The figure shows three views and two pictorial views of one solid part (mm, origin at its lowest corner). Answer the questions. A direction names the side the tool comes from. Give positions to 0.01 mm unless a question says otherwise; leave off trailing zeros. Write each loop counter-clockwise with the first axis right and the second up, starting at its lowest first coordinate (ties: lowest second). Pieces come first, ordered by that corner, then holes. Notation, with made-up numbers: (16.5, 81) -> (62.5, 81) arc R31 cw to (62.5, 110) -> close; hole circle Ø2 at (60, 51.5). An arc over 180 degrees is marked (long way). Write each question's results on one line, items separated by ' | '. Start each with the question number.
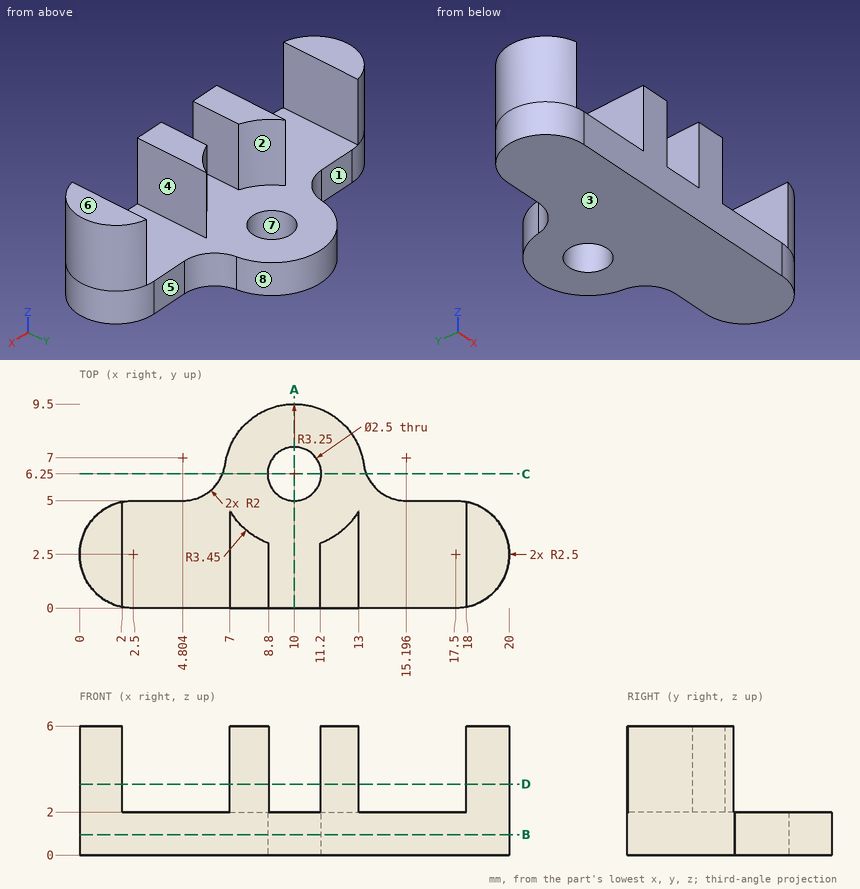
1. The mould has two halves that part along X. Classify the marked faces 6, 7 and 8: pulls with the +X half, pulls with the -X half, needs draft (parallel to the pull), parting line crosses it, or undercut.
2. A tool of negligible diameter and unlimited length cuts with its end or side. For the marked faces 1, 2, 3, 4 and 5, from which of +Z, -Z, +X, -X, +Y, -Y can it reach the whole face along a straight path? Write none if from no direction.
3. Section B-B (z = 0.95) is taken. Write down the section's boundary in (x, y).
4. Each of these flat-tipped pins is pushed along its axis until it touches: pin 1 Ø2.5 at (y, z) = (1, 4) entering from +X; pin 2 Ø1.6 at (x, z) = (16, 1.5) entering from +Y; pin 3 Ø1.2 at (y, z) = (1.5, 4.5) entering from -X. Where does it stop, or does it pass through?
5. Consider probe 1 along Z at (x, y) = (15.5, 3.5); probe 2 along X at (y, z) = (3.5, 0.8). Determine where each line is inside the solid, lowest interval first. Write a range as [from, to].
6. Section C-C (y = 6.25) is taken. Write down the section's boundary in (x, z).
7. Section A-A (x = 10) is taken. Write down the section's boundary in (y, z), then the cut area to 3 significant figures.
8. Section D-D (z = 3.3) is taken. Write down the section's boundary in (x, y).
Results:
1) face 6: needs draft | face 7: undercut | face 8: parting line crosses it
2) face 1: +Z, -Z, -X, +Y | face 2: +Z, +Y | face 3: -Z, +X, -X, +Y, -Y | face 4: +Z, +Y, -Y | face 5: +Z, -Z, +X, +Y
3) outline: (2.5, 0) -> (17.5, 0) arc R2.5 ccw to (17.5, 5) -> (15.2, 5) arc R2 cw to (13.22, 6.71) arc R3.25 ccw to (6.78, 6.71) arc R2 cw to (4.8, 5) -> (2.5, 5) arc R2.5 ccw to start; hole circle Ø2.5 at (10, 6.25)
4) pin 1: stops at x = 19.99 | pin 2: stops at y = 5 | pin 3: stops at x = 0.03
5) probe 1: z = [0, 2] | probe 2: x = [0.21, 19.79]
6) outline: (6.66, 0) -> (8.75, 0) -> (8.75, 2) -> (6.66, 2) -> close; (11.25, 0) -> (13.34, 0) -> (13.34, 2) -> (11.25, 2) -> close
7) outline: (0, 0) -> (5, 0) -> (5, 2) -> (0, 2) -> close; (7.5, 0) -> (9.5, 0) -> (9.5, 2) -> (7.5, 2) -> close | area: 14.0 mm²
8) outline: (2, 0.05) -> (2, 4.95) arc R2.5 ccw to start; (7, 0) -> (8.8, 0) -> (8.8, 3.02) arc R3.45 cw to (7, 4.55) -> close; (11.2, 0) -> (13, 0) -> (13, 4.55) arc R3.45 cw to (11.2, 3.02) -> close; (18, 0.05) arc R2.5 ccw to (18, 4.95) -> close
